from build123d import *

# Parameters (mm, degrees)
BOSS_EXTRUDE1_DEPTH = 35
BOSS_EXTRUDE2_DEPTH = 0.8
SKETCH3_R           = 1.5
BOSS_EXTRUDE3_DEPTH = 0.6
SKETCH5_R           = 1.6
BOSS_EXTRUDE4_DEPTH = 0.6
SKETCH6_W           = 1.996397696
SKETCH6_H           = 1.346407749
SKETCH6_H_2         = 1.346407748
SKETCH6_W_2         = 2.042825549
BOSS_EXTRUDE5_DEPTH = 0.6


with BuildPart() as part:
    # Sketch1 → Boss-Extrude1 (new body)
    with BuildSketch(Plane.XY):
        Polygon((-59.84066795, 5.661190292), (-59.84066795, 7.261190292), (-62.34066795, 7.261190292), (-62.34066795, 9.461190292), (-39.14066795, 9.461190292), (-39.14066795, 7.261190292), (-41.64066795, 7.261190292), (-41.64066795, 5.661190292), (-37.54066795, 5.661190292), (-37.54066795, 11.061190292), (-63.94066795, 11.061190292), (-63.94066795, 5.661190292), align=None)
    extrude(amount=BOSS_EXTRUDE1_DEPTH)

    # Sketch2 → Boss-Extrude2 (add)
    with BuildSketch(Plane(origin=(0, 11.061190292, 0), x_dir=(1, 0, 0), z_dir=(0, 1, 0))):
        with BuildLine():
            Line((-56.64066795, -9.343006494), (-44.84066795, -9.343006494))
            ThreePointArc((-44.84066795, -9.343006494), (-43.34066795, -7.843006494), (-44.84066795, -6.343006494))
            Line((-44.84066795, -6.343006494), (-56.64066795, -6.343006494))
            ThreePointArc((-56.64066795, -6.343006494), (-58.14066795, -7.843006494), (-56.64066795, -9.343006494))
        make_face()
        with BuildLine():
            Line((-58.626258735, -17.853612356), (-42.626258735, -17.853612356))
            ThreePointArc((-42.626258735, -17.853612356), (-41.126258735, -16.353612356), (-42.626258735, -14.853612356))
            Line((-42.626258735, -14.853612356), (-58.626258735, -14.853612356))
            ThreePointArc((-58.626258735, -14.853612356), (-60.126258735, -16.353612356), (-58.626258735, -17.853612356))
        make_face()
        with BuildLine():
            Line((-57.64066795, -28.796277067), (-43.84066795, -28.796277067))
            ThreePointArc((-43.84066795, -28.796277067), (-42.34066795, -27.296277067), (-43.84066795, -25.796277067))
            Line((-43.84066795, -25.796277067), (-57.64066795, -25.796277067))
            ThreePointArc((-57.64066795, -25.796277067), (-59.14066795, -27.296277067), (-57.64066795, -28.796277067))
        make_face()
    extrude(amount=BOSS_EXTRUDE2_DEPTH)

    # Sketch3 → Boss-Extrude3 (add)
    with BuildSketch(Plane.ZY.offset(63.94066795)):
        with Locations((7.526452948, 8.361190292)):
            Circle(SKETCH3_R)
        with Locations((16.495470081, 8.361190292)):
            Circle(SKETCH3_R)
        with Locations((27.258290641, 8.361190292)):
            Circle(SKETCH3_R)
    extrude(amount=BOSS_EXTRUDE3_DEPTH)

    # Sketch5 → Boss-Extrude4 (add)
    with BuildSketch(Plane(origin=(-37.54066795, 0, 0), x_dir=(0, 0, -1), z_dir=(1, 0, 0))):
        with Locations((-27.301707085, 8.361190292)):
            Circle(SKETCH5_R)
        with Locations((-16.305217257, 8.361190292)):
            Circle(SKETCH5_R)
        with Locations((-7.70148216, 8.361190292)):
            Circle(SKETCH5_R)
    extrude(amount=BOSS_EXTRUDE4_DEPTH)

    # Sketch6 → Boss-Extrude5 (add)
    with BuildSketch(Plane.XZ.offset(-5.661190292)):
        with Locations((-39.381913502, 23.535620941)):
            Rectangle(SKETCH6_W, SKETCH6_H)
        with Locations((-61.713710985, 23.883829842)):
            Rectangle(SKETCH6_W, SKETCH6_H_2)
        with Locations((-61.713710985, 19.008905236)):
            Rectangle(SKETCH6_W, SKETCH6_H)
        with Locations((-61.713710985, 13.576846388)):
            Rectangle(SKETCH6_W, SKETCH6_H_2)
        with Locations((-61.690497059, 9.584050996)):
            Rectangle(SKETCH6_W_2, SKETCH6_H_2)
        with Locations((-39.381913502, 18.660696335)):
            Rectangle(SKETCH6_W, SKETCH6_H_2)
        with Locations((-39.381913502, 13.228637488)):
            Rectangle(SKETCH6_W, SKETCH6_H)
        with Locations((-39.358699576, 9.235842096)):
            Rectangle(SKETCH6_W_2, SKETCH6_H)
    extrude(amount=BOSS_EXTRUDE5_DEPTH)


solid = part.part
Verification items for the finished model (mm, model axes). A direction names the side the tool comes from. Coordinates: 2 decimals unless noted, no trailing zeros. Order: outer loops, then holes, each group sorted by start corner. A loop starts at its lowest first (then second) coordinate and runs counter-clockwise, first axis right, second up. Notation, with made-up numbers: M 42.25,69 L 90.25,69 A20 cw 90.25,74 Z; hole C 19,53.25 d11. An arc over 180 degrees is marked long. One line per item, written item: value. Start each with the question number.
Item 1: Gauge pin test, flat ends, axial feed: pin 1 (2 mm diameter, centred on y = 11, z = 21.5, fed in from -X); pin 2 (0.6 mm diameter, centred on x = -52.5, y = 11.5, fed in from +Z); pin 3 (6 mm diameter, centred on x = -43, z = 3.5, fed in from -Y). Record the tip position at first contact, or that the pin passes through.
Item 2: Access from +Z, -Z, +X, -X, +Y, -Y to the whole of each face (thin tool, end or side, straight path). Record for faces 1 (the flat face through (-50.7, 11.5, 17.854)), 2 (the cylindrical face through (-37.245, 7.748, 14.827)), 3 (the cylindrical face through (-58.14, 11.46, 7.81)), 4 (the cylindrical face through (-41.127, 11.456, 16.387)).
Item 3: Sectioned sample at A-A (y = 6.25). Enter the section's corners in (x, z).
Item 4: Sectioned sample at B-B (x = -49). Enter the section's corners in (y, z), then the cut area to 3 significant figures.
Item 5: Scan lines: probe 1 along Z at (x, y) = (-54.25, 11.75); probe 2 along X at (y, z) = (8.5, 7.5); probe 3 along X at (y, z) = (8, 30.5). Record each from-to range of solid material in increasing order.
Item 6: Mould release check, pull along Z, two halves, no side actions. Record for faces 5 (the flat face through (-39, 5.061, 9)), 6 (the cylindrical face through (-64.236, 8.812, 8.957)), 7 (the flat face through (-50.8, 11.5, 28.796)): released by +Z, released by -Z, zero draft, split by the parting line, or undercut.
Item 7: Sectioned sample at C-C (z = 11). Enter the section's corners in (x, y), then the cut area to 3 significant figures.
Conclusion:
1. pin 1: stops at x = -63.94
1. pin 2: stops at z = 28.8
1. pin 3: stops at y = 5.66
2. face 1: +X, -X, +Y
2. face 2: +X
2. face 3: -X, +Y
2. face 4: +X, +Y
3. outline: M -63.94,0 L -59.84,0 L -59.84,35 L -63.94,35 Z; M -41.64,0 L -37.54,0 L -37.54,35 L -41.64,35 Z
4. outline: M 9.46,0 L 11.06,0 L 11.06,6.34 L 11.86,6.34 L 11.86,9.34 L 11.06,9.34 L 11.06,14.85 L 11.86,14.85 L 11.86,17.85 L 11.06,17.85 L 11.06,25.8 L 11.86,25.8 L 11.86,28.8 L 11.06,28.8 L 11.06,35 L 9.46,35 Z
4. area: 63.2 mm^2
5. probe 1: z = 6.34 to 9.34, 14.85 to 17.85, 25.8 to 28.8
5. probe 2: x = -64.54 to -62.34, -39.14 to -36.94
5. probe 3: x = -63.94 to -62.34, -39.14 to -37.54
6. face 5: zero draft
6. face 6: undercut
6. face 7: released by +Z
7. outline: M -63.94,5.66 L -59.84,5.66 L -59.84,7.26 L -62.34,7.26 L -62.34,9.46 L -39.14,9.46 L -39.14,7.26 L -41.64,7.26 L -41.64,5.66 L -37.54,5.66 L -37.54,11.06 L -63.94,11.06 Z
7. area: 62.4 mm^2
